Source: three-view drawing plus pictorial views. Frame: mm from the lowest corner of the part. Give positions to 0.01 mm unless a question says otherwise; leave off trailing zeros. Write each loop counter-clockwise with the first axis right and the second up, starting at its lowest first coordinate (ties: lowest second). Pieces come first, ordered by that corner, then holes. Notation, with made-up numbers: (66.5, 60.25) -> (120.5, 60.25) arc R24 ccw to (120.5, 78.25) -> close; hole circle Ø7 at (-9.5, 57.25). An arc over 180 degrees is marked (long way). Answer in a Markdown table with one row per item. Add a question column.
Item 1: First-contact query: P1, Ø5, axis at x = 100.5, y = 5, coming from the +Z side; P2, Ø5, axis at x = 282.5, y = 4, coming from the +Z side. Flat tips, straight axial feed; report the tip coordinate or a pass-through.
Item 2: Section query A-A on y = 9.5. Output: boundary loops of the cut face in (x, z), plus the area to 3 significant figures.
Item 3: Material intervals for probe 1 along X at (y, z) = (11.5, 164) (1 decimal); probe 2 along Z at (x, y) = (126.5, 5.75) (1 decimal); probe 3 along Z at (x, y) = (209, 8.25), sorted ascending. Write a range as from..to.
Item 4: Section query C-C on x = 311. Output: boundary loops of the cut face in (y, z), plus the area to 3 significant figures.
Item 5: Section query B-B on z = 153.5. Output: boundary loops of the cut face in (x, y), plus the area to 3 significant figures.
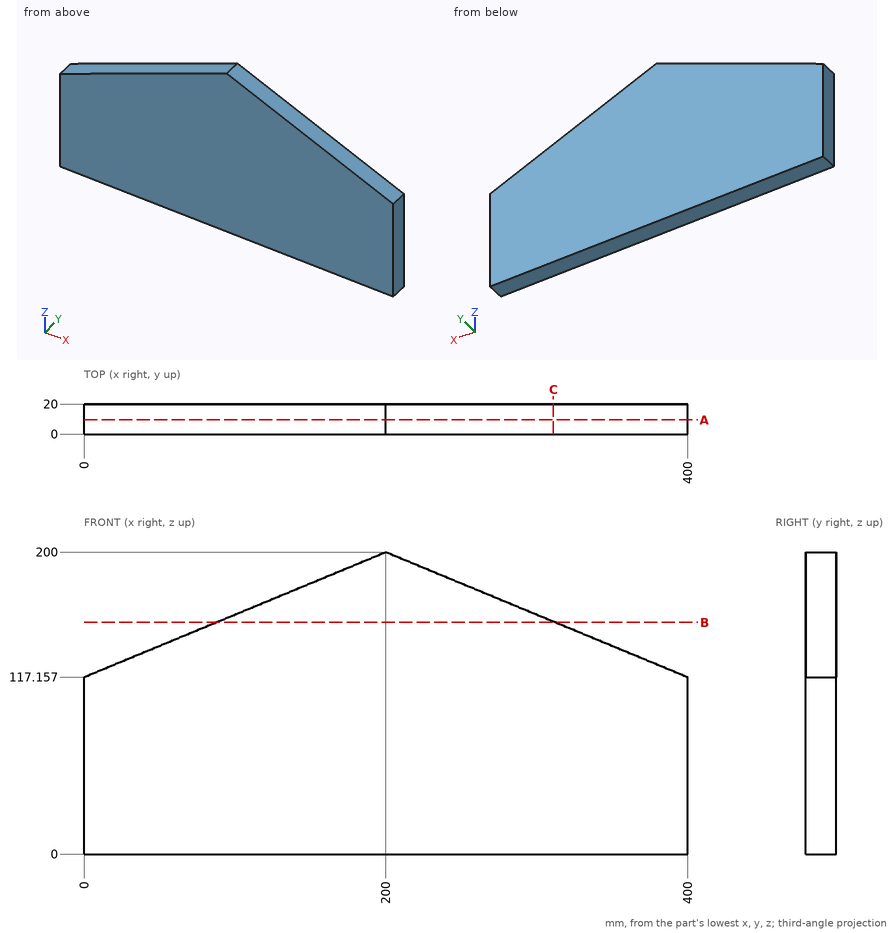
Findings below:
| question | item | result |
|---|---|---|
| 1 | P1 | stops at z = 159.82 |
| 1 | P2 | stops at z = 166.86 |
| 2 | outline | (0, 0) -> (400, 0) -> (400, 117.16) -> (200, 200) -> (0, 117.16) -> close |
| 2 | area | 63,400 mm^2 |
| 3 | probe 1 | x = 113.1..286.9 |
| 3 | probe 2 | z = 0..169.6 |
| 3 | probe 3 | z = 0..196.27 |
| 4 | outline | (0, 0) -> (20, 0) -> (20, 154.02) -> (0, 154.02) -> close |
| 4 | area | 3,080 mm^2 |
| 5 | outline | (87.74, 0) -> (312.26, 0) -> (312.26, 20) -> (87.74, 20) -> close |
| 5 | area | 4,490 mm^2 |
